Verification items for the finished model (mm, model axes). Face numbers are marked on the shaded views. A direction names the side the tool comes from. Give positions to 0.01 mm unless a question says otherwise; leave off trailing zeros. Order: outer loops, then holes, each group sorted by start corner. A loop starts at its lowest first (then second) coordinate and runs counter-clockwise, first axis right, second up.
from build123d import *

# Parameters (mm, degrees)
SKETCH011_R        = 10
PAD008_DEPTH       = 2
SKETCH012_R        = 4.5
PAD009_DEPTH       = 2.5
SKETCH013_R        = 2
POCKET003_DEPTH    = 4.501
CHAMFER004_SIZE    = 0.5
FILLET011_R        = 0.5
SKETCH014_R        = 1.5
POCKET004_DEPTH    = 59.281014
POLARPATTERN_COUNT = 4


with BuildPart() as part:
    # Sketch011 → Pad008 (new body)
    with BuildSketch(Plane.XY):
        Circle(SKETCH011_R)
    extrude(amount=PAD008_DEPTH)

    # Sketch012 (on Face2 of Pad008) → Pad009 (join)
    with BuildSketch(Plane(origin=(0, 0, 0), x_dir=(1, 0, 0), z_dir=(0, 0, -1))):
        Circle(SKETCH012_R)
    extrude(amount=PAD009_DEPTH)

    # Sketch013 (on Face5 of Pad009) → Pocket003 (cut, through all)
    with BuildSketch(Plane(origin=(0, 0, -2.5), x_dir=(1, 0, 0), z_dir=(0, 0, -1))):
        Circle(SKETCH013_R)
    extrude(amount=-POCKET003_DEPTH, mode=Mode.SUBTRACT)

    # Chamfer004
    chamfer004_edges = [part.edges().sort_by_distance(p)[0] for p in [
        (-2, 0, -2.5),
    ]]
    chamfer(chamfer004_edges, length=CHAMFER004_SIZE)

    # Fillet011
    fillet011_edges = [part.edges().sort_by_distance(p)[0] for p in [
        (-4.5, 0, -2.5),
    ]]
    fillet(fillet011_edges, radius=FILLET011_R)

    # Sketch014 (on Face6 of Fillet011) → Pocket004 (cut, through all)
    with BuildSketch(Plane(origin=(0, 0, 0), x_dir=(1, 0, 0), z_dir=(0, 0, -1))):
        with Locations((7, 0)):
            Circle(SKETCH014_R)
    pocket004 = extrude(amount=-POCKET004_DEPTH, mode=Mode.SUBTRACT)

    # PolarPattern: Pocket004 ×4 about axis
    polarpattern_axis = Axis((0, 0, 0), (0, 0, -1))
    for i in range(1, POLARPATTERN_COUNT):
        add(pocket004.rotate(polarpattern_axis, i * 360 / POLARPATTERN_COUNT), mode=Mode.SUBTRACT)


solid = part.part
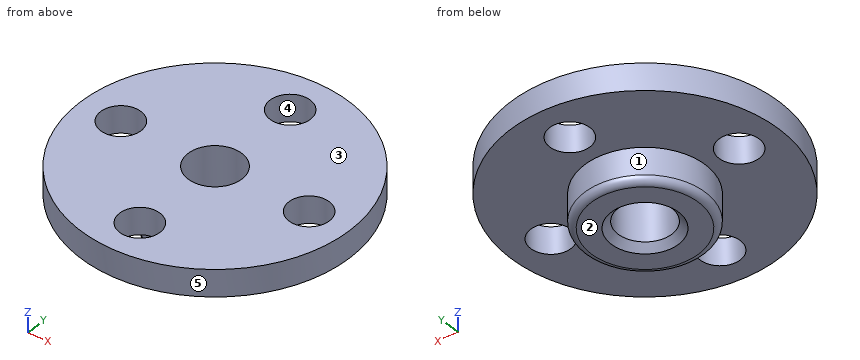
(1) Section check A-A, the plane y = 0. Enter the section's corners in (x, z).
Solved:
outline: (-10, 0) - (-8.5, 0) - (-8.5, 2) - (-10, 2) - close; (-5.5, 0) - (-4.5, 0) - (-4.5, -2) arc R0.5 ccw to (-4, -2.5) - (-2.5, -2.5) - (-2, -2) - (-2, 2) - (-5.5, 2) - close; (2, -2) - (2.5, -2.5) - (4, -2.5) arc R0.5 ccw to (4.5, -2) - (4.5, 0) - (5.5, 0) - (5.5, 2) - (2, 2) - close; (8.5, 0) - (10, 0) - (10, 2) - (8.5, 2) - close
(2) Set-up check for the marked faces 1 and 2: record each of +Z, -Z, +X, -X, +Y, -Y from which the full face is reachable in a straight line by a thin tool's end or side.
Solved:
face 1: -Z
face 2: -Z, +X, -X, +Y, -Y
(3) Release check for a two-part mould opening along Y. For the marked faces 3, 4 and 5 record: pulls with the +Y half, pulls with the -Y half, needs draft (parallel to the pull), parting line crosses it, or undercut.
Solved:
face 3: needs draft
face 4: undercut
face 5: parting line crosses it
(4) Section check C-C, the plane z = 0.25. Enter the section's corners in (x, y).
Solved:
outline: circle Ø20 at (0, 0); hole circle Ø3 at (-7, 0); hole circle Ø4 at (0, 0); hole circle Ø3 at (0, -7); hole circle Ø3 at (0, 7); hole circle Ø3 at (7, 0)
(5) Go/stop test with flat-tipped pins: pin 1 (1.5 mm diameter, centred on x = 5.5, y = -5.5, fed in from -Z); pin 2 (1.5 mm diameter, centred on y = 6, z = -0.5, fed in from -X); pin 3 (3.5 mm diameter, centred on x = 7, y = 0, fed in from +Z). Record where each tip stops, or that it passes through.
Solved:
pin 1: stops at z = 0
pin 2: stops at x = -8.39
pin 3: stops at z = 2
(6) Scan lines: line 1 (Y direction, x = 0, z = -0.9); line 2 (X direction, y = -6, z = 1.4); line 3 (Z direction, x = -3.25, y = -5.5). Record each from-to range of solid material in increasing order.
Solved:
line 1: y = -4.5 to -2, 2 to 4.5
line 2: x = -8 to -1.12, 1.12 to 8
line 3: z = 0 to 2
(7) Section check D-D, the plane x = 7. Enter the section's corners in (y, z), then the cut area to 3 significant figures.
Solved:
outline: (-7.14, 0) - (-1.5, 0) - (-1.5, 2) - (-7.14, 2) - close; (1.5, 0) - (7.14, 0) - (7.14, 2) - (1.5, 2) - close
area: 22.6 mm2
